Can you work these out from the model? Positions are in its coordinate system, mm. A direction names the side the tool comes from. Round coordinates to 2 decimals unless told otherwise and drop trailing zeros. Write each loop counter-clockwise with the first axis right and the second up, starting at its lowest first coordinate (ties: lowest second). Pieces come first, ordered by that corner, then holes.
Q1. Please list where these lines run through material, in increasing order: line 1 along X through (y, z) = (-0.5, -7); line 2 along Y through (x, z) = (16, -12.5); line 3 along Z through (x, y) = (11.5, 2.25).
Q2. If we section it at D-D (x = 13): Please give me the cut outline in (y, z).
Q3. If we section it at C-C (y = 0.75): Please give me the cut outline in (x, z).
Q4. If we section it at B-B (x = 3.5): Please give me the cut outline in (y, z), plus the area to 3 significant figures.
Q5. If we section it at A-A (z = -15): Please give me the cut outline in (x, y).
Q6. I'm going to push flat-ended pins straight in: pin 1 Ø1.3 at (x, y) = (9.5, -1) entering from -Z; pin 2 Ø2 at (x, z) = (8.5, -23.5) entering from +Y; pin 3 Ø1.5 at (x, y) = (13.5, 2) entering from -Z. Where does each tip first touch, or does it pass through?
Q7. For faces 4 (the flat face through (9, 5, -1)), 5 (the flat face through (9, -2, -34)), 6 (the flat face through (17.464, -1, -5)), which set-ups out of +Z, -Z, +X, -X, +Y, -Y let a thin tool reach every point of the face, with its end or its side?
Q8. We'd pull the mould along X, two halves only. Please class faces 1 (the flat face through (9, -4.1, -19)), 2 (the flat face through (2.53, -1, -16)), 3 (the flat face through (0, -3, -17)): +X half, -X half, draft (parallel to the pull), parting line (faces both ways), or undercut.
from build123d import *

# Parameters (mm, degrees)
EXTRUDE_1_DEPTH     = 19.06
CUT_EXTRUDE_1_DEPTH = 2.6
SKETCH_3_W          = 19.06
SKETCH_3_H          = 1.9
EXTRUDE_2_DEPTH     = 5
CUT_EXTRUDE_2_REACH = 41.731
SKETCH_4_W          = 1.8
SKETCH_4_H          = 2
SKETCH_5_W          = 0.5
SKETCH_5_H          = 5
CUT_EXTRUDE_3_DEPTH = 40.730763899


with BuildPart() as part:
    # 草图1 → 凸台-拉伸1 (new body)
    with BuildSketch(Plane(origin=(0, 0, 0), x_dir=(0, 0, -1), z_dir=(1, 0, 0))):
        with BuildLine():
            Line((0, 0), (0, -1.1))
            ThreePointArc((0, -1.1), (0.878679656, -3.221320344), (3, -4.1))
            Line((3, -4.1), (34.5, -4.1))
            Line((34.5, -4.1), (34.5, 0))
            Line((34.5, 0), (0, 0))
        make_face()
    extrude(amount=EXTRUDE_1_DEPTH)

    # 草图2 → 切除-拉伸1 (cut)
    with BuildSketch(Plane(origin=(0, 0, 0), x_dir=(1, 0, 0), z_dir=(0, 1, 0))):
        Polygon((2.53, 28.05), (12.53, 28.05), (12.53, 6.55), (17.464199463, 6.55), (17.464199463, 4.05), (17.464199463, 3.479016937), (12.53, 3.479016937), (11.977918136, 3.479016937), (11.977918136, 4.05), (2.53, 4.05), align=None)
    extrude(amount=-CUT_EXTRUDE_1_DEPTH, mode=Mode.SUBTRACT)

    # 草图3 → 凸台-拉伸2 (add)
    with BuildSketch(Plane(origin=(0, 0, 0), x_dir=(1, 0, 0), z_dir=(0, 1, 0))):
        with Locations((9.53, 0.95)):
            Rectangle(SKETCH_3_W, SKETCH_3_H)
    extrude(amount=EXTRUDE_2_DEPTH)

    # 草图4 → 切除-拉伸2 (cut, up to next)
    with BuildSketch(Plane.ZY, mode=Mode.PRIVATE) as cut_extrude_2_sk1:
        with Locations((-33.6, -1)):
            Rectangle(SKETCH_4_W, SKETCH_4_H)
    cut_extrude_2_tool1 = extrude(cut_extrude_2_sk1.sketch, amount=-CUT_EXTRUDE_2_REACH, mode=Mode.PRIVATE) & part.part
    add(cut_extrude_2_tool1.solids().sort_by_distance((0, -1, -33.6))[0], mode=Mode.SUBTRACT)

    # 草图5 → 切除-拉伸3 (cut, through all)
    with BuildSketch(Plane(origin=(19.06, 0, 0), x_dir=(0, 0, -1), z_dir=(1, 0, 0))):
        with Locations((1.65, 2.5)):
            Rectangle(SKETCH_5_W, SKETCH_5_H)
    extrude(amount=-CUT_EXTRUDE_3_DEPTH, mode=Mode.SUBTRACT)


solid = part.part
A:
1. line 1: x = 0 to 2.53, 12.53 to 19.06
1. line 2: y = -4.1 to 0
1. line 3: z = -1.4 to 0
2. outline: (-4.1, -34.5) - (-2, -34.5) - (-2, -32.7) - (0, -32.7) - (0, -6.55) - (-2.6, -6.55) - (-2.6, -3.48) - (0, -3.48) - (0, -1.4) - (5, -1.4) - (5, 0) - (-1.1, 0) arc R3 ccw to (-4.1, -3) - close
3. outline: (0, -1.4) - (19.06, -1.4) - (19.06, 0) - (0, 0) - close
4. outline: (-4.1, -34.5) - (-2, -34.5) - (-2, -32.7) - (0, -32.7) - (0, -28.05) - (-2.6, -28.05) - (-2.6, -4.05) - (0, -4.05) - (0, -1.4) - (5, -1.4) - (5, 0) - (-1.1, 0) arc R3 ccw to (-4.1, -3) - close
4. area: 80.5 mm2
5. outline: (0, -4.1) - (19.06, -4.1) - (19.06, 0) - (12.53, 0) - (12.53, -2.6) - (2.53, -2.6) - (2.53, 0) - (0, 0) - close
6. pin 1: stops at z = -32.7
6. pin 2: stops at y = -2.6
6. pin 3: stops at z = -1.4
7. face 4: +Z, -Z, +X, -X, +Y
7. face 5: -Z, +X, -X, +Y
7. face 6: +Y
8. face 1: draft
8. face 2: undercut
8. face 3: -X half
